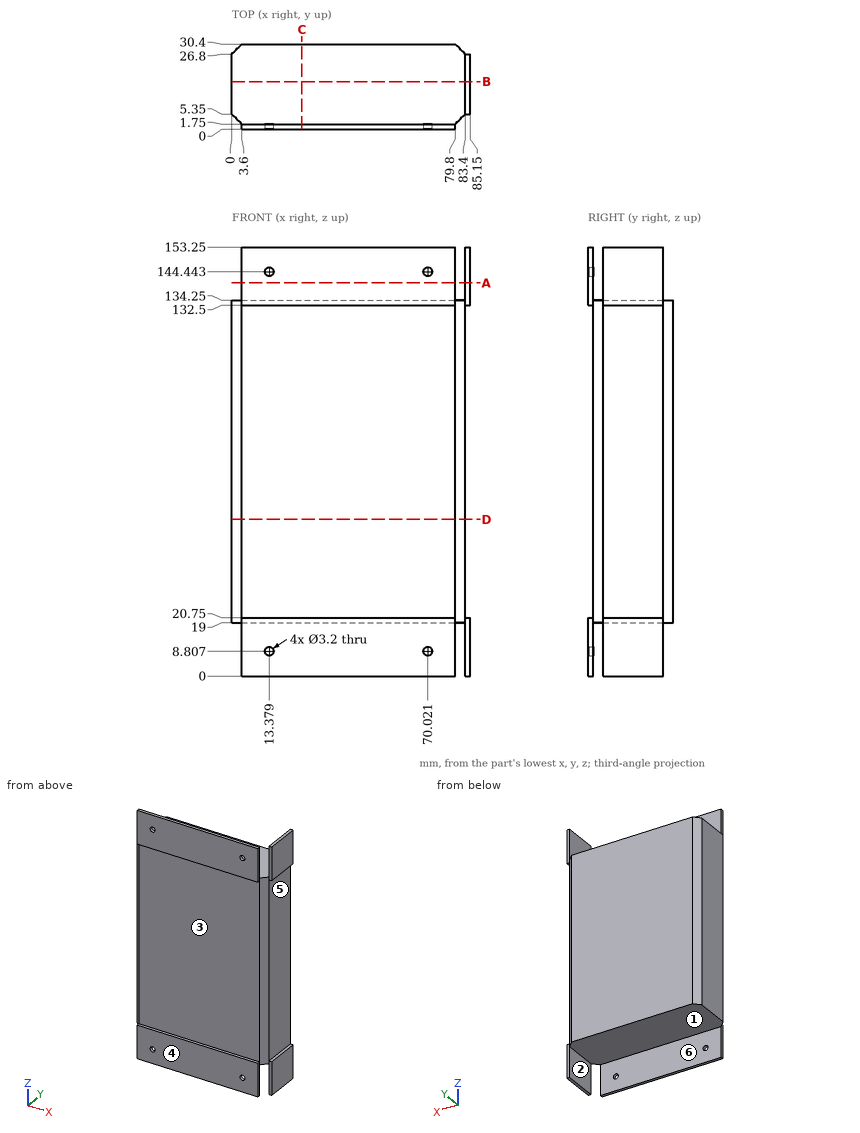
Drawing for the job (mm, zero at the part's lowest x, y, z). A direction names the side the tool comes from. Round coordinates to 2 decimals unless told otherwise and drop trailing zeros. Loops run counter-clockwise (first coordinate to the right, second up) from the corner with the lowest first, then second, coordinate; pieces in that order, holes last. Notation, with made-up numbers: (19, -11.5) -> (53, -11.5) arc R15 ccw to (53, 9.5) -> close; hole circle Ø11 at (81, -28.75). An arc over 180 degrees is marked (long way). Answer as CSV lines item,"result". Start each with the question number.
1) Tool access for the marked faces 4, 5 and 6: list every direction of +Z, -Z, +X, -X, +Y, -Y with a clear straight run to the whole face (end or side of a thin tool).
2) Mould opens along Z. For the marked faces 1, 2 and 3 say: +Z half, -Z half, draft (parallel to the pull), parting line (faces both ways), or undercut.
3) Slice it at B-B (y = 17). List the corners of the cut face in (x, z).
4) Pin check, flat tips, straight feed: P1, Ø9.5, axis at y = 16, z = 8.5, coming from the -X side; P2, Ø1.4, axis at y = 0.5, z = 141, coming from the +X side; P3, Ø14.5, axis at x = 31.5, y = 15.5, coming from the +Z side; P4, Ø1.5, axis at y = 15.5, z = 115.5, coming from the -X side. Stop position of each tip, or through.
5) Slice it at A-A (z = 140.5). List the corners of the cut face in (x, y), plus the area to 3 significant figures.
6) Slice it at D-D (z = 56). List the corners of the cut face in (x, y), plus the area to 3 significant figures.
7) Probe line 1 along Y through (x, z) = (37.5, 113.5); line 2 along X through (y, z) = (19.5, 129); line 3 along Y through (x, z) = (52.5, 9.5). List the from-to ranges inside material, lowest first.
8) Slice it at C-C (x = 25). List the corners of the cut face in (y, z), plus the area to 3 significant figures.
Filled in:
1,face 4,"+Z, -Z, +X, -X, -Y"
1,face 5,"+X, +Y, -Y"
1,face 6,"-Z, +X, -X, +Y"
2,face 1,"-Z half"
2,face 2,"draft"
2,face 3,"undercut"
3,outline,"(0, 19) -> (83.4, 19) -> (83.4, 0) -> (85.15, 0) -> (85.15, 20.75) -> (83.4, 20.75) -> (83.4, 132.5) -> (85.15, 132.5) -> (85.15, 153.25) -> (83.4, 153.25) -> (83.4, 134.25) -> (0, 134.25) -> close"
4,P1,"stops at x = 83.4"
4,P2,"stops at x = 79.8"
4,P3,"stops at z = 134.25"
4,P4,"stops at x = 0"
5,outline,"(3.6, 0) -> (79.8, 0) -> (79.8, 1.75) -> (3.6, 1.75) -> close; (83.4, 5.35) -> (85.15, 5.35) -> (85.15, 26.8) -> (83.4, 26.8) -> close"
5,area,"171 mm2"
6,outline,"(0, 5.35) -> (3.6, 1.75) -> (79.8, 1.75) -> (83.4, 5.35) -> (83.4, 26.8) -> (79.8, 30.4) -> (3.6, 30.4) -> (0, 26.8) -> close"
6,area,"2,360 mm2"
7,line 1,"y = 1.75 to 30.4"
7,line 2,"x = 0 to 83.4"
7,line 3,"y = 0 to 1.75"
8,outline,"(0, 0) -> (1.75, 0) -> (1.75, 19) -> (30.4, 19) -> (30.4, 134.25) -> (1.75, 134.25) -> (1.75, 153.25) -> (0, 153.25) -> (0, 132.5) -> (1.75, 132.5) -> (1.75, 20.75) -> (0, 20.75) -> close"
8,area,"3,370 mm2"
